The model under review builds one solid part; all positions refer to its coordinate system, in mm. A direction names the side the tool comes from. Round coordinates to 2 decimals unless told otherwise and drop trailing zeros. Order: outer loops, then holes, each group sorted by start corner. A loop starts at its lowest first (then second) coordinate and runs counter-clockwise, first axis right, second up. Notation, with made-up numbers: (75.5, 76) -> (80.5, 76) arc R8 ccw to (80.5, 88) -> close; hole circle Ø8 at (-17.75, 37.25). An arc over 180 degrees is marked (long way). Put each result on its own line as item: value. Start each with the question number.
from build123d import *

# Parameters (mm, degrees)
BOSS_EXTRU_1_DEPTH         = 5
ESQUISSE2_W                = 12
ESQUISSE2_H                = 5
ENL_V_MAT_EXTRU_1_DEPTH    = 5
R_P_TITION_LIN_AIRE1_COUNT = 2
R_P_TITION_LIN_AIRE1_PITCH = 24
ESQUISSE4_W                = 5
ESQUISSE4_H                = 13
ENL_V_MAT_EXTRU_2_DEPTH    = 5
R_P_TITION_LIN_AIRE2_COUNT = 3
R_P_TITION_LIN_AIRE2_PITCH = 26
SYM_TRIE1_COPY_1_SKETCH_W  = 5
SYM_TRIE1_COPY_1_SKETCH_H  = 13
SYM_TRIE1_COPY_1_DEPTH     = 5
SYM_TRIE1_COPY_2_SKETCH_W  = 5
SYM_TRIE1_COPY_2_SKETCH_H  = 13
SYM_TRIE1_COPY_2_DEPTH     = 5
BOSS_EXTRU_3_DEPTH         = 5
ESQUISSE7_W                = 20
ESQUISSE7_H                = 5
ENL_V_MAT_EXTRU_3_DEPTH    = 5
ESQUISSE8_W                = 5
ESQUISSE8_H                = 20
ENL_V_MAT_EXTRU_4_DEPTH    = 5


with BuildPart() as part:
    # Esquisse1 → Boss.-Extru.1 (new body)
    with BuildSketch(Plane(origin=(0, 0, 0), x_dir=(0, 0, -1), z_dir=(1, 0, 0))):
        Polygon((0, 0), (0, 35), (45, 35), (45, 0), (60, 0), (60, -65), (0, -65), align=None)
    extrude(amount=BOSS_EXTRU_1_DEPTH)

    # Esquisse2 → Enlèv. mat.-Extru.1 (cut)
    with BuildSketch(Plane(origin=(5, 0, 0), x_dir=(0, 0, -1), z_dir=(1, 0, 0))):
        with Locations((18, -62.5)):
            Rectangle(ESQUISSE2_W, ESQUISSE2_H)
    enl_v_mat_extru_1 = extrude(amount=-ENL_V_MAT_EXTRU_1_DEPTH, mode=Mode.SUBTRACT)

    # Répétition linéaire1: Enlèv. mat.-Extru.1 ×2
    with Locations(*[(0, 0, -i * R_P_TITION_LIN_AIRE1_PITCH) for i in range(1, R_P_TITION_LIN_AIRE1_COUNT)]):
        add(enl_v_mat_extru_1, mode=Mode.SUBTRACT)

    # Esquisse4 → Enlèv. mat.-Extru.2 (cut)
    with BuildSketch(Plane(origin=(5, 0, 0), x_dir=(0, 0, -1), z_dir=(1, 0, 0))):
        with Locations((2.5, -58.5)):
            Rectangle(ESQUISSE4_W, ESQUISSE4_H)
    enl_v_mat_extru_2 = extrude(amount=-ENL_V_MAT_EXTRU_2_DEPTH, mode=Mode.SUBTRACT)

    # Répétition linéaire2: Enlèv. mat.-Extru.2 ×3
    with Locations(*[(0, i * R_P_TITION_LIN_AIRE2_PITCH, 0) for i in range(1, R_P_TITION_LIN_AIRE2_COUNT)]):
        add(enl_v_mat_extru_2, mode=Mode.SUBTRACT)

    # Symétrie1: Enlèv. mat.-Extru.2 across plane
    add(enl_v_mat_extru_2.mirror(Plane.XY.offset(-30)), mode=Mode.SUBTRACT)

    # Symétrie1 copy 1 sketch → Symétrie1 copy 1 (cut)
    with BuildSketch(Plane(origin=(5, 26, -60), x_dir=(0, 0, 1), z_dir=(1, 0, 0))):
        with Locations((2.5, 58.5)):
            Rectangle(SYM_TRIE1_COPY_1_SKETCH_W, SYM_TRIE1_COPY_1_SKETCH_H)
    extrude(amount=-SYM_TRIE1_COPY_1_DEPTH, mode=Mode.SUBTRACT)

    # Symétrie1 copy 2 sketch → Symétrie1 copy 2 (cut)
    with BuildSketch(Plane(origin=(5, 52, -60), x_dir=(0, 0, 1), z_dir=(1, 0, 0))):
        with Locations((2.5, 58.5)):
            Rectangle(SYM_TRIE1_COPY_2_SKETCH_W, SYM_TRIE1_COPY_2_SKETCH_H)
    extrude(amount=-SYM_TRIE1_COPY_2_DEPTH, mode=Mode.SUBTRACT)

    # Esquisse5 → Boss.-Extru.3 (add)
    with BuildSketch(Plane(origin=(5, 0, 0), x_dir=(0, 0, -1), z_dir=(1, 0, 0))):
        Polygon((45, 0), (60, 0), (60, -65), (80, -65), (80, 35), (45, 35), align=None)
    extrude(amount=-BOSS_EXTRU_3_DEPTH)

    # Esquisse7 → Enlèv. mat.-Extru.3 (cut)
    with BuildSketch(Plane(origin=(5, 0, 0), x_dir=(0, 0, -1), z_dir=(1, 0, 0))):
        with Locations((20, 27.5)):
            Rectangle(ESQUISSE7_W, ESQUISSE7_H)
        with Locations((60, 27.5)):
            Rectangle(ESQUISSE7_W, ESQUISSE7_H)
    extrude(amount=-ENL_V_MAT_EXTRU_3_DEPTH, mode=Mode.SUBTRACT)

    # Esquisse8 → Enlèv. mat.-Extru.4 (cut)
    with BuildSketch(Plane(origin=(5, 0, 0), x_dir=(0, 0, -1), z_dir=(1, 0, 0))):
        with Locations((72.5, 5)):
            Rectangle(ESQUISSE8_W, ESQUISSE8_H)
        with Locations((72.5, -35)):
            Rectangle(ESQUISSE8_W, ESQUISSE8_H)
    extrude(amount=-ENL_V_MAT_EXTRU_4_DEPTH, mode=Mode.SUBTRACT)


solid = part.part
Q1. Take a section at C-C on z = -17.5. Give the boundary of the cut face in (x, y), and give its area (3 significant figures).
Q2. Draft analysis for pull direction Z (two halves, no side actions). For faces 1 (the face through (3, -63, -48)), 2 (the face through (3, -25, -72)), 3 (the face through (2, -19, 0)), 4 (the face through (3, -39, -2)), state which applies: +Z half, -Z half, draft (parallel to the pull), parting line (faces both ways), or undercut.
Q3. Take a section at A-A on y = 27.5. Give the boundary of the cut face in (x, z), and give its area (3 significant figures).
Q4. Take a section at B-B on y = 3. Give the boundary of the cut face in (x, z).
Q5. For faces 5 (the face through (3, -59, -5)), 6 (the face through (2, -65, -52)), 7 (the face through (3, 30, -60)), 8 (the face through (3, -63, -36)), 9 (the face through (3, -13, -2)), list the 3-axis set-ups (+Z, -Z, +X, -X, +Y, -Y) from which the entire face can be reached by the end or side of a thin tool; tool diameter is ignored.
Q6. Wall thickness on probe 1 along Z at (x, y) = (4.7, -3); probe 2 along Z at (x, y) = (2.15, 26); probe 3 along Z at (x, y) = (3.4, -56): over which ranges is each line inside the solid? List them lowest first. Write a range as [from, to].
Q7. Clearance check with flat-ended pins moving along their axes: pin 1 Ø2.5 at (x, y) = (3, -59.5) entering from +Z; pin 2 Ø1.5 at (x, z) = (3.5, -57) entering from -Y. State where each tip first meets the part, or that it passes through.
Q8. Take a section at D-D on x = 1. State how many separate pieces and enclosed holes the cut face has, and give its area (3 significant figures).
Calculated:
1. outline: (0, -60) -> (5, -60) -> (5, 25) -> (0, 25) -> close; (0, 30) -> (5, 30) -> (5, 35) -> (0, 35) -> close
1. area: 450 mm²
2. face 1: undercut
2. face 2: undercut
2. face 3: +Z half
2. face 4: draft
3. outline: (0, -80) -> (5, -80) -> (5, -70) -> (0, -70) -> close; (0, -50) -> (5, -50) -> (5, -30) -> (0, -30) -> close; (0, -10) -> (5, -10) -> (5, 0) -> (0, 0) -> close
3. area: 200 mm²
4. outline: (0, -80) -> (5, -80) -> (5, -75) -> (0, -75) -> close; (0, -70) -> (5, -70) -> (5, 0) -> (0, 0) -> close
5. face 5: +Z, +X, -X, -Y
5. face 6: +Z, -Z, +X, -X, -Y
5. face 7: +X, -X
5. face 8: +X, -X, -Y
5. face 9: +Z, +X, -X
6. probe 1: z = [-80, -75], [-70, -60], [-55, -5]
6. probe 2: z = [-80, -70], [-50, -30], [-10, 0]
6. probe 3: z = [-80, -60], [-55, -5]
7. pin 1: stops at z = -5
7. pin 2: stops at y = -52
8. separate pieces: 1
8. enclosed holes: 6
8. area: 7,090 mm²
